Input: part model. Units: mm. Frame: model coordinates. A direction names the side the tool comes from. Coordinates: 2 decimals unless noted, no trailing zeros. Loops run counter-clockwise (first coordinate to the right, second up) from the corner with the lowest first, then second, coordinate; pieces in that order, holes last. Notation, with made-up numbers: M 19.25,31 L 43.25,31 A20 ccw 43.25,69 Z; hole C 32,70.5 d10. An arc over 180 degrees is marked long. Use a Markdown table: item, result. Add a question column.
1. Line query: L1, parallel to X at y = 10.75, z = -3.9; L2, parallel to Y at x = 0, z = -4; L3, parallel to Z at x = -17.5, y = 10. Output: solid intervals per line, ascending. Write a range as [from, to].
2. Section B-B on y = 15. Output: boundary loops of the cut face in (x, z).
3. Section A-A on z = 0. Output: boundary loops of the cut face in (x, y).
4. Pin query (flat end, axial travel): pin 1 (6.5 mm diameter, centred on x = 2, y = 12, fed in from +Z); pin 2 (5.5 mm diameter, centred on x = 0, y = 15, fed in from +Z) (3 decimals); pin 3 (14.5 mm diameter, centred on x = 0, y = 15, fed in from -Z). Return the tip coordinate at first contact, or that it passes through.
5. Draft query along Y for faces 3 (the cylindrical face through (-6.4, 9.6, -3.6)), 4 (the cylindrical face through (19.1, 16.3, 1.2)), 5 (the flat face through (0, 30, 0)), 6 (the cylindrical face through (7.3, 9.25, -3.58)). Return one class per face: +Y half, -Y half, draft (parallel to the pull), parting line (faces both ways), or undercut.
6. Set-up query: faces 1 (the flat face through (-5, 25, 5)), 2 (the cylindrical face through (-0.82, 21.246, -2.841)). Return all of +Z, -Z, +X, -X, +Y, -Y with unobstructed straight access to the full face (end or side cutting, diameter ignored); none if empty.
7. Section D-D on y = 10.75. Output: boundary loops of the cut face in (x, z), then the cut area to 3 significant figures.
8. Section C-C on x = 17.5. Output: boundary loops of the cut face in (y, z).
Autodesk Inventor part; units mm, degrees
ref_plane "YZ Plane" through (0, 0, 0) normal (1, 0, 0) x (0, 1, 0)
ref_plane "XZ Plane" through (0, 0, 0) normal (0, 1, 0) x (-1, 0, 0)
ref_plane "XY Plane" through (0, 0, 0) normal (0, 0, 1) x (1, 0, 0)
sketch "Sketch1" plane through (0, 0, 0) normal (0, 1, 0) x (-1, 0, 0)
  line L0 (22.5, 5) -> (-22.5, 5)
  line L1 (-22.5, 5) -> (-22.5, -5)
  line L2 (-22.5, -5) -> (22.5, -5)
  line L3 (22.5, -5) -> (22.5, 5)
  line L4 (22.5, 5) -> (-22.5, -5) construction
  line L5 (-22.5, 5) -> (22.5, -5) construction
  line L6 (0, 0) -> (17.5, 0) construction
  line L7 (0, 0) -> (-17.5, 0) construction
  circle A0 centre (17.5, 0) radius 2
  circle A1 centre (-17.5, 0) radius 2
  line L8 (22.5, 5) -> (17.5, 5)
  line L9 (17.5, 5) -> (17.5, 0) construction
  dimension "d0" = 45
  dimension "d1" = 10
  dimension "d2" = 17.5
  dimension "d3" = 17.5
  dimension "d4" = 4
  dimension "d5" = 4
extrude "Extrusion1" add sketch "Sketch1" along normal blind 30
sketch "Sketch2" plane through (0, 0, 0) normal (0, -1, 0) x (1, 0, 0)
  line L0 (-22.5, -5) -> (-22.5, 5)
  line L1 (22.5, -5) -> (-22.5, -5)
  line L2 (-22.5, 5) -> (22.5, 5)
  line L3 (22.5, 5) -> (22.5, -5)
  line L4 (22.5, -5) -> (-22.5, -5)
  line L5 (-22.5, -5) -> (-22.5, 5)
  circle A0 centre (-17.5, 0) radius 2
  circle A1 centre (-17.5, 0) radius 1.6
  circle A2 centre (17.5, 0) radius 2
  circle A3 centre (17.5, 0) radius 1.6
sketch "Sketch3" plane through (-22.5, 0, 5) normal (0, 0, 1) x (1, 0, 0)
  line L0 (45, 30) -> (0, 30) construction
  line L1 (0, 30) -> (45, 0) construction
  line L2 (45, 0) -> (0, 0) construction
  line L3 (45, 30) -> (0, 0) construction
  circle A0 centre (22.5, 15) radius 3
  circle A1 centre (22.5, 15) radius 7.5 construction
  circle A2 centre (22.5, 22.5) radius 1.1
  circle A3 centre (16.0048, 11.25) radius 1.1
  circle A4 centre (28.9952, 11.25) radius 1.1
  point P0 (22.5, 0)
  dimension "d9" = 15
  dimension "d8" = 6
  dimension "d10" = 2.2
  dimension "d13" = 360
extrude "Extrusion2" cut sketch "Sketch3" against normal blind 30 contours A0
sketch "Sketch4" plane through (-22.5, 0, 5) normal (0, 0, 1) x (1, 0, 0)
  line L0 (45, 0) -> (45, 30) construction
  line L1 (0, 30) -> (45, 0) construction
  line L2 (45, 30) -> (0, 30) construction
  line L3 (0, 0) -> (45, 30) construction
  circle A0 centre (22.5, 15) radius 6.3
  point P0 (22.5, 0)
  dimension "d17" = 12.6
extrude "Extrusion3" cut sketch "Sketch4" against normal blind 8.5
sketch "Sketch5" plane through (-22.5, 0, 5) normal (0, 0, 1) x (1, 0, 0)
  line L0 (0, 0) -> (0, 30) construction
  line L1 (0, 0) -> (45, 0) construction
  line L2 (0, 30) -> (45, 0) construction
  line L3 (0, 30) -> (45, 30) construction
  line L4 (45, 30) -> (0, 0) construction
  circle A0 centre (22.5, 15) radius 11
  point P0 (22.5, 0)
  dimension "d20" = 22
extrude "Extrusion4" cut sketch "Sketch5" against normal blind 7.2
extrude "Extrusion5" cut sketch "Sketch2" against normal blind 3 contours L0 L2 L3 L1
sketch "Sketch6" plane through (22.5, 30, -5) normal (0, 0, -1) x (-1, 0, 0)
  circle A0 centre (22.5, -15) radius 3
  circle A1 centre (22.5, -15) radius 8.5 construction
  point P0 (22.5, -30)
  point P1 (22.5, -6.5)
  point P2 (15.1388, -19.25)
  point P3 (29.8612, -19.25)
  dimension "d25" = 17
  dimension "d28" = 360
hole "Bohrung2" at (0, 15, -5) at (7.3612, 10.75, -5) at (-7.3612, 10.75, -5) at (0, 23.5, -5) direction (0, 0, 1) diameter 3 end through all
properties part number "MotorBracket"
Answers below:
| question | item | result |
|---|---|---|
| 1 | L1 | x = [-22.5, -8.86], [-5.86, 5.86], [8.86, 22.5] |
| 1 | L2 | y = [3, 12], [18, 22], [25, 30] |
| 1 | L3 | z = [-5, -2], [2, 5] |
| 2 | outline | M -22.5,-5 L -3,-5 L -3,-3.5 L -6.3,-3.5 L -6.3,-2.2 L -11,-2.2 L -11,5 L -22.5,5 Z; M 3,-5 L 22.5,-5 L 22.5,5 L 11,5 L 11,-2.2 L 6.3,-2.2 L 6.3,-3.5 L 3,-3.5 Z; hole C -17.5,0 d4; hole C 17.5,0 d4 |
| 3 | outline | M -22.5,3 L -19.5,3 L -19.5,30 L -22.5,30 Z; M -15.5,3 L 15.5,3 L 15.5,30 L -15.5,30 Z; M 19.5,3 L 22.5,3 L 22.5,30 L 19.5,30 Z; hole C 0,15 d22 |
| 4 | pin 1 | stops at z = -2.2 |
| 4 | pin 2 | passes through |
| 4 | pin 3 | stops at z = -5 |
| 5 | face 3 | undercut |
| 5 | face 4 | draft |
| 5 | face 5 | +Y half |
| 5 | face 6 | undercut |
| 6 | face 1 | +Z, +X, -X, +Y, -Y |
| 6 | face 2 | +Z |
| 7 | outline | M -22.5,-5 L -8.86,-5 L -8.86,-2.2 L -10.15,-2.2 L -10.15,5 L -22.5,5 Z; M -5.86,-5 L 5.86,-5 L 5.86,-2.2 L 4.65,-2.2 L 4.65,-3.5 L -4.65,-3.5 L -4.65,-2.2 L -5.86,-2.2 Z; M 8.86,-5 L 22.5,-5 L 22.5,5 L 10.15,5 L 10.15,-2.2 L 8.86,-2.2 Z; hole C -17.5,0 d4; hole C 17.5,0 d4 |
| 7 | area | 250 mm² |
| 8 | outline | M 3,-5 L 30,-5 L 30,-2 L 3,-2 Z; M 3,2 L 30,2 L 30,5 L 3,5 Z |
